```python
from build123d import *

# Parameters (mm, degrees)
CUT_EXTRUDE1_DEPTH = 0.91


with BuildPart() as part:
    # Sketch2 → Revolve1 (revolve)
    with BuildSketch(Plane(origin=(0, 0, 0), x_dir=(0, 0, -1), z_dir=(1, 0, 0)), mode=Mode.PRIVATE) as revolve1_sk:
        with BuildLine():
            Line((-3.15, 0), (3.15, 0))
            Line((3.15, 0), (3.15, 0.68))
            Line((3.15, 0.68), (2.83, 1))
            Line((2.83, 1), (-1.85, 1))
            Line((-1.85, 1), (-1.85, 1.75))
            Line((-1.85, 1.75), (-2.045, 1.75))
            ThreePointArc((-2.045, 1.75), (-2.670023043, 1.481850617), (-3.15, 1))
            Line((-3.15, 1), (-3.15, 0))
        make_face()
    revolve(revolve1_sk.sketch.rotate(Axis((0, 0, 3.15), (0, 0, -1)), 90), axis=Axis((0, 0, 3.15), (0, 0, -1)))

    # Sketch3 → Cut-Extrude1 (cut)
    with BuildSketch(Plane.XY.offset(3.15)):
        Polygon((0, 0.75055535), (-0.65, 0.375277675), (-0.65, -0.375277675), (0, -0.75055535), (0.65, -0.375277675), (0.65, 0.375277675), align=None)
    extrude(amount=-CUT_EXTRUDE1_DEPTH, mode=Mode.SUBTRACT)

    # Cut-Extrude2 cone 1 section (through the dimple's axis) → Cut-Extrude2 (revolve, cut)
    with BuildSketch(Plane(origin=(0, 0, 3.15), x_dir=(0, -1, 0), z_dir=(1, 0, 0))):
        Polygon((0, 0), (0.75055535, 0), (0, 0.75055535), align=None)
    revolve(axis=Axis((0, 0, 3.15), (0, 0, -1)), mode=Mode.SUBTRACT)


solid = part.part
```
Part model, mm, in its own coordinate system. Round coordinates to 2 decimals unless told otherwise and drop trailing zeros. Order: outer loops, then holes, each group sorted by start corner. A loop starts at its lowest first (then second) coordinate and runs counter-clockwise, first axis right, second up. Notation, with made-up numbers: M 36.25,40 L 73.25,40 A29 cw 73.25,71 Z; hole C -32,18 d1. An arc over 180 degrees is marked long. Answer in a Markdown table with one row per item. Add a question column.
Q1. Cut at B-B on z = 2.5. Give the cut face in (x, y), and give its area (3 significant figures).
Q2. Cut at D-D on x = -1.35. Give the cut face in (y, z) (3 decimals), and give its area (3 significant figures).
Q3. Pin check, flat tips, straight feed: pin 1 (1.5 mm diameter, centred on x = -1, z = -2, fed in from +Y); pin 2 (1 mm diameter, centred on x = -1, z = 1, fed in from +Y); pin 3 (1.5 mm diameter, centred on x = -1, z = -2, fed in from -Y). Stop position of each tip, or through.
Q4. Cut at A-A on y = 0. Give the cut face in (x, z) (3 decimals).
Q5. Mould opens along X. For faces 1 (the face through (0, 1, 0)), 2 (the face through (0, 0, 2.24)), 3 (the face through (0, 0, -3.15)) say: +X half, -X half, draft (parallel to the pull), parting line (faces both ways), or undercut.
Q6. Cut at C-C on z = 0. Give the cut face in (x, y), and give its area (3 significant figures).
Q7. Wall check: L1, parallel to X at y = 0.15, z = 3; L2, parallel to Z at x = 1.3, y = -0.65; L3, parallel to Z at x = -0.9, y = 1.2. Give the ranges that are in metal, low to high. Write a range as from..to.
Established:
| question | item | result |
|---|---|---|
| 1 | outline | C 0,0 d3.17; hole M -0.65,-0.38 L 0,-0.75 L 0.65,-0.38 L 0.65,0.38 L 0,0.75 L -0.65,0.38 Z |
| 1 | area | 6.42 mm2 |
| 2 | outline | M -1.114,1.85 L 1.114,1.85 L 1.114,2.045 A1.177 ccw -1.114,2.045 Z |
| 2 | area | 1.73 mm2 |
| 3 | pin 1 | stops at y = 0.97 |
| 3 | pin 2 | stops at y = 0.87 |
| 3 | pin 3 | stops at y = -0.97 |
| 4 | outline | M -1.75,1.85 L -1,1.85 L -1,-2.83 L -0.68,-3.15 L 0.68,-3.15 L 1,-2.83 L 1,1.85 L 1.75,1.85 L 1.75,2.045 A1.791 ccw 1,3.15 L 0.751,3.15 L 0.65,3.049 L 0.65,2.24 L -0.65,2.24 L -0.65,3.049 L -0.751,3.15 L -1,3.15 A1.791 ccw -1.75,2.045 Z |
| 5 | face 1 | parting line |
| 5 | face 2 | undercut |
| 5 | face 3 | draft |
| 6 | outline | C 0,0 d2 |
| 6 | area | 3.14 mm2 |
| 7 | L1 | x = -1.18..-0.65, 0.65..1.18 |
| 7 | L2 | z = 1.85..2.71 |
| 7 | L3 | z = 1.85..2.64 |
